Autodesk Inventor part; units mm, degrees
ref_plane "YZ Plane" through (0, 0, 0) normal (1, 0, 0) x (0, 1, 0)
ref_plane "XZ Plane" through (0, 0, 0) normal (0, 1, 0) x (-1, 0, 0)
ref_plane "XY Plane" through (0, 0, 0) normal (0, 0, 1) x (1, 0, 0)
sketch "Эскиз1" plane through (0, 0, 0) normal (0, 0, 1) x (1, 0, 0)
  line L0 (0, 0) -> (200, 0) construction
  line L1 (10.5713, 250) -> (75.6527, 250) construction
  line L2 (98, 0) -> (102, 0) construction
  line L3 (102, 0) -> (102, 250) construction
  line L4 (98, 250) -> (102, 250) construction
  line L5 (98, 0) -> (98, 250) construction
  line L6 (98, 250) -> (102, 0) construction
  line L7 (0, 127) -> (200, 127)
  line L8 (200, 127) -> (200, 123)
  line L9 (200, 123) -> (0, 123)
  line L10 (0, 123) -> (0, 127)
  line L11 (0, 127) -> (200, 123) construction
  line L12 (200, 127) -> (0, 123) construction
  line L13 (0, 186) -> (200, 186)
  line L14 (200, 186) -> (200, 190)
  line L15 (200, 190) -> (0, 190)
  line L16 (0, 190) -> (0, 186)
  line L17 (0, 0) -> (4, 0)
  line L18 (4, 0) -> (4, 250)
  line L19 (4, 250) -> (0, 250)
  line L20 (0, 250) -> (0, 0)
  line L21 (200, 0) -> (196, 0)
  line L22 (196, 0) -> (196, 250)
  line L23 (196, 250) -> (200, 250)
  line L24 (200, 250) -> (200, 0)
  line L25 (0, 59) -> (200, 59)
  line L26 (200, 59) -> (200, 63)
  line L27 (200, 63) -> (0, 63)
  line L28 (0, 63) -> (0, 59)
  arc A0 (193.3786, 241.9343) -> (189.4287, 250) centre (189.4287, 245) ccw
  arc A1 (10.5713, 250) -> (6.6214, 241.9343) centre (10.5713, 245) ccw
  arc A2 (0, 0) -> (6.6214, 241.9343) centre (-144.0414, 125) ccw
  arc A3 (193.3786, 241.9343) -> (200, 0) centre (344.0414, 125) ccw
  arc A4 (78.2507, 248.5) -> (75.6527, 250) centre (75.6527, 247) ccw
  line L29 (124.3473, 250) -> (189.4287, 250)
  arc A5 (124.3473, 250) -> (121.7493, 248.5) centre (124.3473, 247) ccw
  line L30 (121.7493, 248.5) -> (112.751, 232.9146)
  arc A6 (108.4209, 230.4146) -> (112.751, 232.9146) centre (108.4209, 235.4146) ccw
  line L31 (108.4209, 230.4146) -> (91.5791, 230.4146)
  arc A7 (87.249, 232.9146) -> (91.5791, 230.4146) centre (91.5791, 235.4146) ccw
  line L32 (87.249, 232.9146) -> (78.2507, 248.5)
  point P0 (100, 125)
  point P1 (4, 186)
  point P2 (196, 186)
  point P3 (196, 127)
  point P4 (4, 127)
  point P5 (0, 186)
  point P6 (4, 123)
  point P7 (196, 123)
  point P8 (196, 190)
  point P9 (4, 190)
  point P10 (0, 190)
  point P11 (196, 63)
  point P12 (4, 63)
  point P13 (4, 59)
  point P14 (196, 59)
  dimension "d0" = 200
  dimension "d1" = 4
  dimension "d2" = 200
  dimension "d3" = 4
  dimension "d4" = 4
  dimension "d5" = 250
  dimension "d6" = 4
  dimension "d7" = 250
  dimension "d10" = 60
  dimension "d11" = 200
  dimension "d12" = 4
  dimension "d13" = 60
extrude "Выдавливание1" add sketch "Эскиз1" along normal mid plane 100 contours L20 L13 L18 L7 | L7 L18 L9 L10 | L7 A2 L9 L18 | L9 L18 L27 L20 | L16 L15 L18 L13 | L7 A3 L9 A2 | L18 L15 A2 L13 | L27 L18 L25 L20 | L20 L19 L18 L15 | L7 L22 L9 A3 | A2 L15 A3 L13 | L27 A2 L25 L18 | L25 L18 A2 L20 | L22 L13 L24 L7 | L7 L8 L9 L22 | A3 L15 L22 L13 | L27 A3 L25 A2 | A2 L18 L17 | L9 L24 L27 L22 | L22 L15 L14 L13 | L27 L22 L25 A3 | L27 L24 L25 L22 | L22 L23 L24 L15 | L25 L24 A3 L22 | A3 L21 L22
sketch "Эскиз2" plane through (4, 190, 50) normal (0, 1, 0) x (1, 0, 0)
  line L0 (196, 100) -> (196, 0)
  line L1 (-4, 0) -> (196, 100) construction
  ellipse E0 centre (96, 50) end of major axis (111.5174, 50) minor radius 11
  point P0 (-4, 50)
  dimension "d16" = 11
extrude "Выдавливание2" cut sketch "Эскиз2" against normal blind 300
properties part number "ребра для шкафа"
For this review, take the finished solid that the model builds, in its own axes (mm). A direction names the side the tool comes from. Coordinates: 2 decimals unless noted, no trailing zeros. Order: outer loops, then holes, each group sorted by start corner. A loop starts at its lowest first (then second) coordinate and runs counter-clockwise, first axis right, second up. Notation, with made-up numbers: (-7.75, 0.5) - (2.25, 0.5) arc R11 cw to (2.25, 16.5) - close; hole circle Ø1 at (-6, 65). An arc over 180 degrees is marked (long way). Answer as CSV lines item,"result". Start each with the question number.
1) Machinability: for faces 5 (the flat face through (101, 123, -12)), 6 (the flat face through (101, 190, -12)), 7 (the flat face through (4, 29, -1)), which of the approach directions +Z, -Z, +X, -X, +Y, -Y give a long, thin tool a straight path to every point of the face, cutting with its end or side? Answer none if there is none.
2) Insertion check: P1, Ø18, axis at y = 87.5, z = 13.5, coming from the -X side; P2, Ø6, axis at x = 96.5, z = 20, coming from the -Y side; P3, Ø8, axis at x = 80, z = -10, coming from the +Y side. Each pin has a flat end and moves straight along its axis. Give the tip position at first contact, or say it passes through.
3) Add section B-B (y = 196). State the section outline as (x, z) points.
4) To check wall thickness, follow line 1 along Y through (x, z) = (128.5, -1); line 2 along X through (y, z) = (28, 24). State the ranges of each line that lie inside material, in increasing order. Write a range as [from, to].
5) Add section A-A (x = 143). State the section outline as (y, z) points.
6) Add section C-C (z = 16). State the section outline as (x, y) points.
7) Draft analysis for pull direction Y (two halves, no side actions). For faces 1 (the flat face through (196, 156, -1)), 2 (the flat face through (99, 59, -12)), 3 (the flat face through (4, 220, -1)), 4 (the flat face through (99, 127, -12)), state which applies: +Y half, -Y half, draft (parallel to the pull), parting line (faces both ways), or undercut.
Result:
1,face 5,"+Z, -Z"
1,face 6,"+Z, -Z, +Y"
1,face 7,"+Z, -Z, -Y"
2,P1,"x = 0"
2,P2,"y = 59"
2,P3,"y = 190"
3,outline,"(0, -50) - (4, -50) - (4, 50) - (0, 50) - close; (196, -50) - (200, -50) - (200, 50) - (196, 50) - close"
4,line 1,"[59, 63], [123, 127], [186, 190]"
4,line 2,"[0, 4], [196, 200]"
5,outline,"(59, -50) - (63, -50) - (63, 50) - (59, 50) - close; (123, -50) - (127, -50) - (127, 50) - (123, 50) - close; (186, -50) - (190, -50) - (190, 50) - (186, 50) - close"
6,outline,"(0, 0) - (4, 0) - (4, 59) - (196, 59) - (196, 0) - (200, 0) - (200, 250) - (196, 250) - (196, 190) - (4, 190) - (4, 250) - (0, 250) - close; hole (4, 63) - (196, 63) - (196, 123) - (4, 123) - close; hole (4, 127) - (196, 127) - (196, 186) - (4, 186) - close"
7,face 1,"undercut"
7,face 2,"-Y half"
7,face 3,"draft"
7,face 4,"undercut"
